Verification items for this drawing (mm, ordinates from the low corner). Round coordinates to 2 decimals unless told otherwise and drop trailing zeros. Order: outer loops, then holes, each group sorted by start corner. A loop starts at its lowest first (then second) coordinate and runs counter-clockwise, first axis right, second up. Notation, with made-up numbers: (5, 25) -> (23, 25) arc R20 cw to (23, 30) -> close; hole circle Ø1 at (-39.5, 47.25). An arc over 180 degrees is marked (long way). Answer in a Markdown table with one row per item.
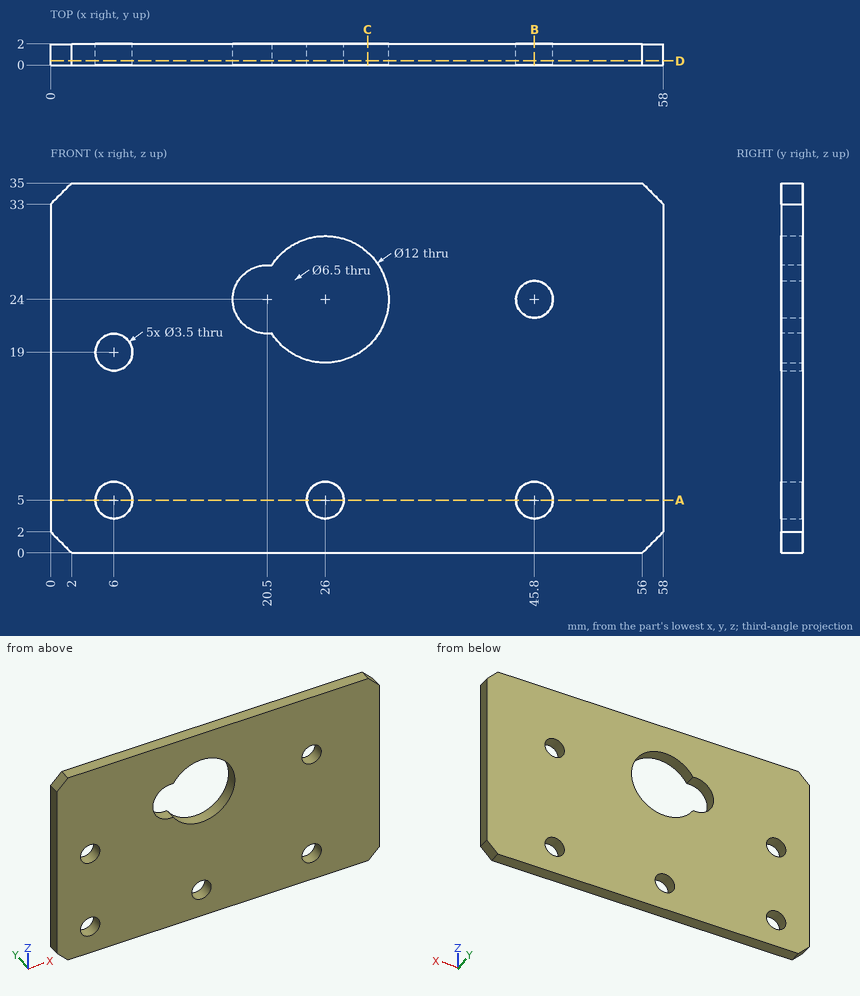
Item 1: Depth check by flat-ended pin: P1, Ø9.5, axis at x = 26, z = 24, coming from the +Y side. Enter the tip coordinate at first touch or a pass-through.
Result sheet:
| item | result |
|---|---|
| P1 | passes through |
Item 2: Cross-section at D-D (y = 0.4). Record the boundary of the cut face in (x, z), and give its area (3 significant figures).
Result sheet:
| item | result |
|---|---|
| outline | (0, 2) -> (2, 0) -> (56, 0) -> (58, 2) -> (58, 33) -> (56, 35) -> (2, 35) -> (0, 33) -> close; hole circle Ø3.5 at (6, 5); hole circle Ø3.5 at (6, 19); hole (20.94, 20.78) arc R6 ccw (long way) to (20.94, 27.22) arc R3.25 ccw (long way) to start; hole circle Ø3.5 at (26, 5); hole circle Ø3.5 at (45.8, 5); hole circle Ø3.5 at (45.8, 24) |
| area | 1,850 mm^2 |
Item 3: Cross-section at B-B (x = 45.8). Record the boundary of the cut face in (y, z), and give its area (3 significant figures).
Result sheet:
| item | result |
|---|---|
| outline | (0, 0) -> (2, 0) -> (2, 3.25) -> (0, 3.25) -> close; (0, 6.75) -> (2, 6.75) -> (2, 22.25) -> (0, 22.25) -> close; (0, 25.75) -> (2, 25.75) -> (2, 35) -> (0, 35) -> close |
| area | 56.0 mm^2 |
Item 4: Cross-section at C-C (x = 30). Record the boundary of the cut face in (y, z), and give its area (3 significant figures).
Result sheet:
| item | result |
|---|---|
| outline | (0, 0) -> (2, 0) -> (2, 19.53) -> (0, 19.53) -> close; (0, 28.47) -> (2, 28.47) -> (2, 35) -> (0, 35) -> close |
| area | 52.1 mm^2 |
Item 5: Scan lines: line 1 (X direction, y = 1, z = 5); line 2 (Z direction, x = 26, y = 1.1); line 3 (X direction, y = 1.3, z = 19). Record each from-to range of solid material in increasing order. Write a range as [from, to].
Result sheet:
| item | result |
|---|---|
| line 1 | x = [0, 4.25], [7.75, 24.25], [27.75, 44.05], [47.55, 58] |
| line 2 | z = [0, 3.25], [6.75, 18], [30, 35] |
| line 3 | x = [0, 4.25], [7.75, 22.68], [29.32, 58] |
Item 6: Cross-section at A-A (z = 5). Record the boundary of the cut face in (x, y).
Result sheet:
| item | result |
|---|---|
| outline | (0, 0) -> (4.25, 0) -> (4.25, 2) -> (0, 2) -> close; (7.75, 0) -> (24.25, 0) -> (24.25, 2) -> (7.75, 2) -> close; (27.75, 0) -> (44.05, 0) -> (44.05, 2) -> (27.75, 2) -> close; (47.55, 0) -> (58, 0) -> (58, 2) -> (47.55, 2) -> close |
